from build123d import *

# Parameters (mm, degrees)
SKETCH1_W           = 61
SKETCH1_H           = 79.25
BOSS_EXTRUDE1_DEPTH = 3.5
SKETCH2_R           = 1.5
CUT_EXTRUDE1_DEPTH  = 3.5
FILLET1_R           = 3
SKETCH3_R           = 1.5
CUT_EXTRUDE2_DEPTH  = 3.5


with BuildPart() as part:
    # Sketch1 → Boss-Extrude1 (new body)
    with BuildSketch(Plane(origin=(0, 0, 0), x_dir=(1, 0, 0), z_dir=(0, 1, 0))):
        Rectangle(SKETCH1_W, SKETCH1_H)
    extrude(amount=BOSS_EXTRUDE1_DEPTH)

    # Sketch2 → Cut-Extrude1 (cut)
    with BuildSketch(Plane(origin=(0, 3.5, 0), x_dir=(1, 0, 0), z_dir=(0, 1, 0))):
        with Locations(Location((-27.5, 36.625, 0), (0, 0, 270))):
            Circle(SKETCH2_R)
        with Locations(Location((27.5, 36.625, 0), (0, 0, 270))):
            Circle(SKETCH2_R)
        with Locations(Location((-27.5, -36.625, 0), (0, 0, 270))):
            Circle(SKETCH2_R)
        with Locations(Location((27.5, -36.625, 0), (0, 0, 270))):
            Circle(SKETCH2_R)
    extrude(amount=-CUT_EXTRUDE1_DEPTH, mode=Mode.SUBTRACT)

    # Fillet1
    fillet1_edges = [part.edges().sort_by_distance(p)[0] for p in [
        (30.5, 1.75, 39.625),
        (-30.5, 1.75, 39.625),
        (-30.5, 1.75, -39.625),
        (30.5, 1.75, -39.625),
    ]]
    fillet(fillet1_edges, radius=FILLET1_R)

    # Sketch3 → Cut-Extrude2 (cut)
    with BuildSketch(Plane(origin=(0, 3.5, 0), x_dir=(1, 0, 0), z_dir=(0, 1, 0))):
        with Locations(Location((-24.5, -22.125, 0), (0, 0, 270))):
            Circle(SKETCH3_R)
        with Locations(Location((24.5, -22.125, 0), (0, 0, 270))):
            Circle(SKETCH3_R)
        with Locations(Location((19.5, 28.375, 0), (0, 0, 270))):
            Circle(SKETCH3_R)
        with Locations(Location((-8.5, 28.375, 0), (0, 0, 270))):
            Circle(SKETCH3_R)
    extrude(amount=-CUT_EXTRUDE2_DEPTH, mode=Mode.SUBTRACT)


solid = part.part
For this review, take the finished solid that the model builds, in its own axes (mm). Coordinates: 2 decimals unless noted, no trailing zeros. Loops run counter-clockwise (first coordinate to the right, second up) from the corner with the lowest first, then second, coordinate; pieces in that order, holes last. Notation, with made-up numbers: (88, 77) -> (119, 77) arc R20 cw to (119, 89) -> close; hole circle Ø3 at (-11.5, 30.5). An arc over 180 degrees is marked (long way). Write each question's results on one line, items separated by ' | '.
Q1. To check wall thickness, follow line 1 along Z through (x, y) = (25, 1.4) (3 decimals); line 2 along Z through (x, y) = (-9.5, 0.9) (3 decimals). State the ranges of each line that lie inside material, in increasing order. Write a range as [from, to].
Taken from the geometry:
line 1: [-39.625, 20.711], [23.539, 39.625] | line 2: [-39.625, -29.493], [-27.257, 39.625]
Q2. For pin 1 Ø2.5 at (x, z) = (-24.5, 22.125) entering from -Y, flat-tipped, find the tip position at first contact; note if it passes through.
Taken from the geometry:
pin 1: through
Q3. Add section A-A, the plane x = 19.5. State the section outline as (y, z) points (3 decimals).
Taken from the geometry:
outline: (0, -39.625) -> (3.5, -39.625) -> (3.5, -29.875) -> (0, -29.875) -> close; (0, -26.875) -> (3.5, -26.875) -> (3.5, 39.625) -> (0, 39.625) -> close
Q4. Mouldability with a two-part tool opening along Z and no side actions: class faces 1 (the cylindrical face through (-29.645, 1.774, -38.723)), 2 (the flat face through (-30.5, 2, 1)), 3 (the cylindrical face through (-23.486, 1.774, 21.019)), 4 (the cylindrical face through (28.987, 1.774, -36.82)) as +Z half, -Z half, draft (parallel to the pull), parting line (faces both ways), or undercut.
Taken from the geometry:
face 1: -Z half | face 2: draft | face 3: undercut | face 4: undercut
